Autodesk Inventor part; units mm, degrees
ref_plane "YZ Plane" through (0, 0, 0) normal (1, 0, 0) x (0, 1, 0)
ref_plane "XZ Plane" through (0, 0, 0) normal (0, 1, 0) x (-1, 0, 0)
ref_plane "XY Plane" through (0, 0, 0) normal (0, 0, 1) x (1, 0, 0)
sketch "Boceto1" plane through (0, 0, 0) normal (0, 1, 0) x (-1, 0, 0)
  line L0 (140, 75) -> (-140, 75)
  line L1 (-200, 15) -> (-200, -15)
  line L2 (-140, -75) -> (140, -75)
  arc A0 (-140, 75) -> (-200, 15) centre (-140, 15) ccw
  arc A1 (-200, -15) -> (-140, -75) centre (-140, -15) ccw
  line L3 (-140, 65) -> (-140, 55)
  line L4 (-140, -55) -> (-140, -65)
  arc A2 (-140, 65) -> (-190, 15) centre (-140, 15) ccw
  line L5 (-190, 15) -> (-190, -15)
  arc A3 (-190, -15) -> (-140, -65) centre (-140, -15) ccw
  arc A4 (-140, 55) -> (-180, 15) centre (-140, 15) ccw
  line L6 (-180, 15) -> (-180, -15)
  arc A5 (-180, -15) -> (-140, -55) centre (-140, -15) ccw
  line L7 (140, 65) -> (140, 55)
  line L8 (140, -55) -> (140, -65)
  arc A6 (190, 15) -> (140, 65) centre (140, 15) ccw
  line L9 (190, 15) -> (190, -15)
  arc A7 (140, -65) -> (190, -15) centre (140, -15) ccw
  arc A8 (180, 15) -> (140, 55) centre (140, 15) ccw
  line L10 (180, 15) -> (180, -15)
  arc A9 (140, -55) -> (180, -15) centre (140, -15) ccw
  line L11 (200, 15) -> (200, -15)
  arc A10 (200, 15) -> (140, 75) centre (140, 15) ccw
  arc A11 (140, -75) -> (200, -15) centre (140, -15) ccw
  circle A12 centre (0, 0) radius 10
  dimension "d32" = 400
  dimension "d33" = 150
extrude "Extrusión1" add sketch "Boceto1" along normal blind 15 contours A6 L9 A7 L8 A9 L10 A8 L7
extrude "Extrusión2" add sketch "Boceto1" along normal blind 15 contours L3 A4 L6 A5 L4 A3 L5 A2
extrude "Extrusión3" add sketch "Boceto1" along normal blind 30
extrude "Extrusión4" add sketch "Boceto1" along normal blind 10 contours A12
hole "Agujero1" at (0, 0, 0) direction (0, 1, 0) diameter 3 end through all
properties part number "base"
The model under review builds one solid part; all positions refer to its coordinate system, in mm. A direction names the side the tool comes from. Give positions to 0.01 mm unless a question says otherwise; leave off trailing zeros. Order: outer loops, then holes, each group sorted by start corner. A loop starts at its lowest first (then second) coordinate and runs counter-clockwise, first axis right, second up. Notation, with made-up numbers: M 0.25,39 L 40.25,39 A22 ccw 40.25,48 Z; hole C 7.25,87.5 d7. An arc over 180 degrees is marked long. Use one line per item in the form item = value. Start each with the question number.
Item 1: For faces 4 (the cylindrical face through (-181.96, 14.79, 57.89)), 5 (the cylindrical face through (174.964, 22.395, -50.742)), list the 3-axis set-ups (+Z, -Z, +X, -X, +Y, -Y) from which the entire face can be reached by the end or side of a thin tool; tool diameter is ignored.
Item 2: The part is to be moulded in two halves that separate along Z. For faces 1 (the cylindrical face through (-182.89, 14.79, -56.96)), 2 (the flat face through (3, 30, 18)), 3 (the cylindrical face through (-168.594, 22.395, -42.972)), say which applies: pulls with the +Z half, pulls with the -Z half, needs draft (parallel to the pull), parting line crosses it, or undercut.
Item 3: Insertion check: pin 1 Ø10 at (x, z) = (1.5, 3) entering from +Y; pin 2 Ø8 at (y, z) = (20, 57.5) entering from -X; pin 3 Ø11 at (y, z) = (24, 62) entering from +X; pin 4 Ø2.5 at (x, z) = (0, 0) entering from +Y. Each pin has a flat end and moves straight along its axis. Give the tip position at first contact, or say it passes through.
Item 4: We need section C-C on z = -39. Give the boundary of the cut face in (x, y), plus the area to 3 significant figures.
Item 5: We need section A-A on y = 24.5. Give the boundary of the cut face in (x, z), plus the area to 3 significant figures.
Item 6: We need section B-B on y = 3.5. Give the boundary of the cut face in (x, z), plus the area to 3 significant figures.
Item 7: To check wall thickness, follow line 1 along Z through (x, y) = (0, 20); line 2 along X through (y, z) = (18.25, -12); line 3 along X through (y, z) = (8, 0). State the ranges of each line that lie inside material, in increasing order. Write a range as from..to.
Completed:
q1.face_4 = +Z, -X, +Y, -Y
q1.face_5 = +Y
q2.face_1 = pulls with the -Z half
q2.face_2 = needs draft
q2.face_3 = undercut
q3.pin_1 = 10
q3.pin_2 = -186.02
q3.pin_3 = 183.33
q3.pin_4 = through
q4.outline = M -194.99,0 L 194.99,0 L 194.99,30 L 183.86,30 L 183.86,15 L 172,15 L 172,30 L -172,30 L -172,15 L -183.86,15 L -183.86,30 L -194.99,30 Z
q4.area = 11,300 mm²
q5.outline = M -200,-15 A60 ccw -140,-75 L 140,-75 A60 ccw 200,-15 L 200,15 A60 ccw 140,75 L -140,75 A60 ccw -200,15 Z; hole M -190,-15 A50 ccw -140,-65 L -140,-55 A40 cw -180,-15 L -180,15 A40 cw -140,55 L -140,65 A50 ccw -190,15 Z; hole C 0,0 d20; hole M 140,-65 A50 ccw 190,-15 L 190,15 A50 ccw 140,65 L 140,55 A40 cw 180,15 L 180,-15 A40 cw 140,-55 Z
q5.area = 53,200 mm²
q6.outline = M -200,-15 A60 ccw -140,-75 L 140,-75 A60 ccw 200,-15 L 200,15 A60 ccw 140,75 L -140,75 A60 ccw -200,15 Z; hole C 0,0 d3
q6.area = 56,900 mm²
q7.line_1 = -75..-10, 10..75
q7.line_2 = -200..-190, -180..180, 190..200
q7.line_3 = -200..-1.5, 1.5..200
